```python
from build123d import *

# Parameters (mm, degrees)
SKETCH_1_W                = 48.5
SKETCH_1_H                = 37
EXTRUDE_1_DEPTH           = 3
SKETCH_2_W                = 21.920667416
SKETCH_2_H                = 2.787
CUT_EXTRUDE_1_DEPTH       = 32.646484797
SKETCH_6_W                = 21.920667416
SKETCH_6_H                = 2.787
CUT_EXTRUDE_5_DEPTH       = 32.646484797
EXTRUDE_2_DEPTH           = 3.028
EXTRUDE_3_DEPTH           = 3.028
HOLE_WIZARD_M4_1_D        = 4.447
HOLE_WIZARD_3_0_3_1_D     = 3
HOLE_WIZARD_3_0_3_1_DEPTH = 6.028
SKETCH_13_W               = 34.5
SKETCH_13_H               = 26.000497192
CUT_EXTRUDE_7_DEPTH       = 10
CHAMFER_1_SIZE            = 3
SKETCH_14_W               = 3
SKETCH_14_H               = 4
CUT_EXTRUDE_8_DEPTH       = 2
CHAMFER_2_SIZE            = 3
CHAMFER_2_SIZE_2          = 3.981134465
SKETCH_15_W               = 2
SKETCH_15_H               = 3
CUT_EXTRUDE_9_DEPTH       = 1.5
CHAMFER_3_SIZE            = 2


with BuildPart() as part:
    # 草图1 → 凸台-拉伸1 (new body)
    with BuildSketch(Plane.XY.offset(-11)):
        with Locations((1.25, 0)):
            Rectangle(SKETCH_1_W, SKETCH_1_H)
    extrude(amount=-EXTRUDE_1_DEPTH)

    # 草图2 → 切除-拉伸1 (cut, through all)
    with BuildSketch(Plane(origin=(0, 0, -14), x_dir=(-1, 0, 0), z_dir=(0, 0, -1))):
        with Locations((6.539666292, -11.606748596)):
            Rectangle(SKETCH_2_W, SKETCH_2_H)
    extrude(amount=-CUT_EXTRUDE_1_DEPTH, mode=Mode.SUBTRACT)

    # 草图6 → 切除-拉伸5 (cut, through all)
    with BuildSketch(Plane(origin=(0, 0, -14), x_dir=(-1, 0, 0), z_dir=(0, 0, -1))):
        with Locations((6.539666292, 11.606748596)):
            Rectangle(SKETCH_6_W, SKETCH_6_H)
    extrude(amount=-CUT_EXTRUDE_5_DEPTH, mode=Mode.SUBTRACT)

    # 草图7 → 凸台-拉伸2 (add)
    with BuildSketch(Plane.XY.offset(-11)):
        with BuildLine():
            Line((-20.5, -12), (-20.5, 12))
            ThreePointArc((-20.5, 12), (-19.914213562, 13.414213562), (-18.5, 14))
            Line((-18.5, 14), (-18.5, 12.914213562))
            ThreePointArc((-18.5, 12.914213562), (-19.224744871, 12.366025404), (-19.5, 11.5))
            Line((-19.5, 11.5), (-19.5, -11.5))
            ThreePointArc((-19.5, -11.5), (-19.224744871, -12.366025404), (-18.5, -12.914213562))
            Line((-18.5, -12.914213562), (-18.5, -14))
            ThreePointArc((-18.5, -14), (-19.914213562, -13.414213562), (-20.5, -12))
        make_face()
    extrude(amount=EXTRUDE_2_DEPTH)

    # 草图8 → 凸台-拉伸3 (add)
    with BuildSketch(Plane.XY.offset(-11)):
        with BuildLine():
            Line((19.5, -11.5), (19.5, 11.5))
            ThreePointArc((19.5, 11.5), (19.224744871, 12.366025404), (18.5, 12.914213562))
            Line((18.5, 12.914213562), (18.5, 14))
            ThreePointArc((18.5, 14), (19.914213562, 13.414213562), (20.5, 12))
            Line((20.5, 12), (20.5, -12))
            ThreePointArc((20.5, -12), (19.914213562, -13.414213562), (18.5, -14))
            Line((18.5, -14), (18.5, -12.914213562))
            ThreePointArc((18.5, -12.914213562), (19.224744871, -12.366025404), (19.5, -11.5))
        make_face()
    extrude(amount=EXTRUDE_3_DEPTH)

    # M4 间隙孔1 (through all)
    with Locations(Plane.XY.offset(-11)):
        with Locations((12.25, 6.000000304)):
            Hole(HOLE_WIZARD_M4_1_D / 2)

    # Ø3.0 (3) 直径孔1
    with Locations(Plane(origin=(0, 0, -14), x_dir=(-1, 0, 0), z_dir=(0, 0, -1))):
        with Locations((-15, -16.5), (15, -16.5), (0, -16.5), (-15, 16.5), (15, 16.5), (0, 16.5)):
            Hole(HOLE_WIZARD_3_0_3_1_D / 2, depth=HOLE_WIZARD_3_0_3_1_DEPTH)

    # 草图13 → 切除-拉伸7 (cut, symmetric)
    with BuildSketch(Plane(origin=(0, 0, -14), x_dir=(-1, 0, 0), z_dir=(0, 0, -1))):
        with Locations((0.75, 0)):
            Rectangle(SKETCH_13_W, SKETCH_13_H)
    extrude(amount=CUT_EXTRUDE_7_DEPTH, both=True, mode=Mode.SUBTRACT)

    # 倒角1
    chamfer_1_edges = [part.edges().sort_by_distance(p)[0] for p in [
        (-23, 18.5, -12.5),
        (25.5, 18.5, -12.5),
        (25.5, -18.5, -12.5),
        (-23, -18.5, -12.5),
    ]]
    chamfer(chamfer_1_edges, length=CHAMFER_1_SIZE)

    # 草图14 → 切除-拉伸8 (cut)
    with BuildSketch(Plane(origin=(0, 0, -14), x_dir=(-1, 0, 0), z_dir=(0, 0, -1))):
        with Locations((-7.5, -16.5)):
            Rectangle(SKETCH_14_W, SKETCH_14_H)
        with Locations((7.5, -16.5)):
            Rectangle(SKETCH_14_W, SKETCH_14_H)
        with Locations((7.5, 16.5)):
            Rectangle(SKETCH_14_W, SKETCH_14_H)
        with Locations((-7.5, 16.5)):
            Rectangle(SKETCH_14_W, SKETCH_14_H)
    extrude(amount=-CUT_EXTRUDE_8_DEPTH, mode=Mode.SUBTRACT)

    # 倒角2
    # the kernel refuses this chamfer: 3.981134465, 3 mm, written as the material it adds along each edge
    with BuildSketch(Plane(origin=(-6, 14.5, -12), x_dir=(0, -0.04104604510109815, -0.9991572559820394), z_dir=(-1, 0, 0))) as chamfer_2_piece_1_section:
        Polygon((CHAMFER_2_SIZE * 0.999157255982, -CHAMFER_2_SIZE * 0.0410460451011), (-CHAMFER_2_SIZE_2 * 0.0410460450997, -CHAMFER_2_SIZE_2 * 0.999157255947), (0, 0), align=None)
    chamfer_2_piece_1 = extrude(amount=3, mode=Mode.PRIVATE)
    chamfer_2_piece_1 = split(chamfer_2_piece_1, bisect_by=Plane(origin=(-7.5, 15.961237376, -14), z_dir=(0, 0, 1)), keep=Keep.TOP, mode=Mode.PRIVATE)
    add(chamfer_2_piece_1)
    with BuildSketch(Plane(origin=(9, 14.5, -12), x_dir=(0, -0.04104604510109815, -0.9991572559820394), z_dir=(-1, 0, 0))) as chamfer_2_piece_2_section:
        Polygon((CHAMFER_2_SIZE * 0.999157255982, -CHAMFER_2_SIZE * 0.0410460451011), (-CHAMFER_2_SIZE_2 * 0.0410460450997, -CHAMFER_2_SIZE_2 * 0.999157255947), (0, 0), align=None)
    chamfer_2_piece_2 = extrude(amount=3, mode=Mode.PRIVATE)
    chamfer_2_piece_2 = split(chamfer_2_piece_2, bisect_by=Plane(origin=(7.5, 15.961237376, -14), z_dir=(0, 0, 1)), keep=Keep.TOP, mode=Mode.PRIVATE)
    add(chamfer_2_piece_2)
    with BuildSketch(Plane(origin=(-9, -14.5, -12), x_dir=(0, -0.9997280272590685, 0.023321052992758363), z_dir=(1, 0, 0))) as chamfer_2_piece_3_section:
        Polygon((CHAMFER_2_SIZE_2 * 0.999728027224, CHAMFER_2_SIZE_2 * 0.0233210529919), (-CHAMFER_2_SIZE * 0.0233210529928, CHAMFER_2_SIZE * 0.999728027259), (0, 0), align=None)
    chamfer_2_piece_3 = extrude(amount=3, mode=Mode.PRIVATE)
    chamfer_2_piece_3 = split(chamfer_2_piece_3, bisect_by=Plane(origin=(-7.5, -15.961237376, -14), z_dir=(0, 0, 1)), keep=Keep.TOP, mode=Mode.PRIVATE)
    add(chamfer_2_piece_3)
    with BuildSketch(Plane(origin=(6, -14.5, -12), x_dir=(0, -0.9997280272590685, 0.023321052992758374), z_dir=(1, 0, 0))) as chamfer_2_piece_4_section:
        Polygon((CHAMFER_2_SIZE_2 * 0.999728027224, CHAMFER_2_SIZE_2 * 0.0233210529919), (-CHAMFER_2_SIZE * 0.0233210529928, CHAMFER_2_SIZE * 0.999728027259), (0, 0), align=None)
    chamfer_2_piece_4 = extrude(amount=3, mode=Mode.PRIVATE)
    chamfer_2_piece_4 = split(chamfer_2_piece_4, bisect_by=Plane(origin=(7.5, -15.961237376, -14), z_dir=(0, 0, 1)), keep=Keep.TOP, mode=Mode.PRIVATE)
    add(chamfer_2_piece_4)

    # 草图15 → 切除-拉伸9 (cut)
    with BuildSketch(Plane(origin=(0, 0, -14), x_dir=(-1, 0, 0), z_dir=(0, 0, -1))):
        with Locations((-24.5, -9.5)):
            Rectangle(SKETCH_15_W, SKETCH_15_H)
        with Locations((-24.5, 9.5)):
            Rectangle(SKETCH_15_W, SKETCH_15_H)
        with Locations((22, 9.5)):
            Rectangle(SKETCH_15_W, SKETCH_15_H)
        with Locations((22, -9.5)):
            Rectangle(SKETCH_15_W, SKETCH_15_H)
    extrude(amount=-CUT_EXTRUDE_9_DEPTH, mode=Mode.SUBTRACT)

    # 倒角3
    # the kernel refuses this chamfer: 2 mm, written as the material it adds along each edge
    with BuildSketch(Plane(origin=(-21, 2.856634024, -12.5), x_dir=(0.027495876610585623, 0, -0.9996219169112968), z_dir=(0, 1, 0))) as chamfer_3_piece_1_section:
        Polygon((CHAMFER_3_SIZE * 0.999621916911, CHAMFER_3_SIZE * 0.0274958766106), (-CHAMFER_3_SIZE * 0.0274958766106, CHAMFER_3_SIZE * 0.999621916911), (0, 0), align=None)
    chamfer_3_piece_1 = extrude(amount=13.286731952, mode=Mode.PRIVATE)
    chamfer_3_piece_1 = split(chamfer_3_piece_1, bisect_by=Plane(origin=(-21.7, 9.5, -14), z_dir=(0, 0, 1)), keep=Keep.TOP, mode=Mode.PRIVATE)
    chamfer_3_piece_1 = split(chamfer_3_piece_1, bisect_by=Plane(origin=(-25.35, 13.15, -13.1), z_dir=(0.7071067811865476, -0.7071067811865476, 0)), keep=Keep.TOP, mode=Mode.PRIVATE)
    add(chamfer_3_piece_1)
    with BuildSketch(Plane(origin=(-21, -2.856634024, -12.5), x_dir=(0.027495876610585623, 0, -0.9996219169112968), z_dir=(0, -1, 0))) as chamfer_3_piece_2_section:
        Polygon((CHAMFER_3_SIZE * 0.999621916911, -CHAMFER_3_SIZE * 0.0274958766106), (-CHAMFER_3_SIZE * 0.0274958766106, -CHAMFER_3_SIZE * 0.999621916911), (0, 0), align=None)
    chamfer_3_piece_2 = extrude(amount=8.143365976, mode=Mode.PRIVATE)
    chamfer_3_piece_2 = split(chamfer_3_piece_2, bisect_by=Plane(origin=(-21.7, -9.5, -14), z_dir=(0, 0, 1)), keep=Keep.TOP, mode=Mode.PRIVATE)
    add(chamfer_3_piece_2)
    with BuildSketch(Plane(origin=(23.5, 2.856634024, -12.5), x_dir=(-0.027495876610585623, 0, -0.9996219169112968), z_dir=(0, 1, 0))) as chamfer_3_piece_3_section:
        Polygon((CHAMFER_3_SIZE * 0.999621916911, -CHAMFER_3_SIZE * 0.0274958766106), (-CHAMFER_3_SIZE * 0.0274958766106, -CHAMFER_3_SIZE * 0.999621916911), (0, 0), align=None)
    chamfer_3_piece_3 = extrude(amount=8.143365976, mode=Mode.PRIVATE)
    chamfer_3_piece_3 = split(chamfer_3_piece_3, bisect_by=Plane(origin=(24.2, 9.5, -14), z_dir=(0, 0, 1)), keep=Keep.TOP, mode=Mode.PRIVATE)
    add(chamfer_3_piece_3)
    with BuildSketch(Plane(origin=(23.5, -2.856634024, -12.5), x_dir=(-0.027495876610585623, 0, -0.9996219169112968), z_dir=(0, -1, 0))) as chamfer_3_piece_4_section:
        Polygon((CHAMFER_3_SIZE * 0.999621916911, CHAMFER_3_SIZE * 0.0274958766106), (-CHAMFER_3_SIZE * 0.0274958766106, CHAMFER_3_SIZE * 0.999621916911), (0, 0), align=None)
    chamfer_3_piece_4 = extrude(amount=13.286731952, mode=Mode.PRIVATE)
    chamfer_3_piece_4 = split(chamfer_3_piece_4, bisect_by=Plane(origin=(24.2, -9.5, -14), z_dir=(0, 0, 1)), keep=Keep.TOP, mode=Mode.PRIVATE)
    chamfer_3_piece_4 = split(chamfer_3_piece_4, bisect_by=Plane(origin=(27.85, -13.15, -13.1), z_dir=(-0.7071067811865476, 0.7071067811865476, 0)), keep=Keep.TOP, mode=Mode.PRIVATE)
    add(chamfer_3_piece_4)


solid = part.part
```
Part model, mm, in its own coordinate system. A direction names the side the tool comes from. Give positions to 0.01 mm unless a question says otherwise; leave off trailing zeros. Loops run counter-clockwise (first coordinate to the right, second up) from the corner with the lowest first, then second, coordinate; pieces in that order, holes last. Notation, with made-up numbers: M -2,-31 L 28,-31 A24 ccw 28,-7 Z; hole C -32,27.25 d2. An arc over 180 degrees is marked long. Return JSON: item names as keys, results as strings.
1) 3-axis set-ups, long thin cutter, end or side, ignore diameter. For faces 4 (the face through (16.5, 0, -13)), 5 (the face through (24.9, 8, -13.4)), 6 (the face through (18.5, -13.5, -9.5)): which of +Z, -Z, +X, -X, +Y, -Y reach the whole face in a straight line?
Calculated:
{"face 4": "+Z, -Z", "face 5": "-Z, +X", "face 6": "+Z, +Y, -Y"}
2) Pull direction Y, two halves, no side cores. Call faces 1 (the face through (19.9, 13.43, -9.51)), 2 (the face through (-19.5, 0, -10)), 3 (the face through (20.5, 0, -10)): released by +Y, released by -Y, zero draft, split by the parting line, or undercut.
Calculated:
{"face 1": "released by +Y", "face 2": "undercut", "face 3": "zero draft"}
3) Saw through at D-D, the plane y = -16.5. List the corners of the cut face in (x, z).
Calculated:
{"outline": "M -22,-14 L -16.5,-14 L -16.5,-11 L -22,-11 Z; M -13.5,-14 L -9,-14 L -9,-13.49 L -6,-13.49 L -6,-14 L -1.5,-14 L -1.5,-11 L -13.5,-11 Z; M 1.5,-14 L 6,-14 L 6,-13.49 L 9,-13.49 L 9,-14 L 13.5,-14 L 13.5,-11 L 1.5,-11 Z; M 16.5,-14 L 24.5,-14 L 24.5,-11 L 16.5,-11 Z"}
4) Saw through at C-C, the plane z = -10. List the corners of the cut face in (x, y), then the cut area to 3 significant figures.
Calculated:
{"outline": "M -20.5,-12 A2 ccw -18.5,-14 L -18.5,-12.91 A1.5 cw -19.5,-11.5 L -19.5,11.5 A1.5 cw -18.5,12.91 L -18.5,14 A2 ccw -20.5,12 Z; M 18.5,-14 A2 ccw 20.5,-12 L 20.5,12 A2 ccw 18.5,14 L 18.5,12.91 A1.5 cw 19.5,11.5 L 19.5,-11.5 A1.5 cw 18.5,-12.91 Z", "area": "58.4 mm2"}
5) Drill centre lines: line 1 (Y direction, x = 0, z = -12.45); line 2 (X direction, y = 3.5, z = -10.75); line 3 (Y direction, x = -12.5, z = -13.5). Where is each one in solid material? Low to high.
Calculated:
{"line 1": "y = -18.5 to -18, -15 to -13, 13 to 15, 18 to 18.5", "line 2": "x = -20.5 to -19.5, 19.5 to 20.5", "line 3": "y = -18.5 to -13, 13 to 18.5"}
6) Saw through at A-A, the plane y = 6. List the corners of the cut face in (x, z).
Calculated:
{"outline": "M -23,-14 L -18,-14 L -18,-11 L -19.5,-11 L -19.5,-7.97 L -20.5,-7.97 L -20.5,-11 L -23,-11 Z; M 16.5,-14 L 25.5,-14 L 25.5,-11 L 20.5,-11 L 20.5,-7.97 L 19.5,-7.97 L 19.5,-11 L 16.5,-11 Z"}
7) Saw through at B-B, the plane x = -2. List the corners of the cut face in (y, z), then the cut area to 3 significant figures.
Calculated:
{"outline": "M -18.5,-14 L -13,-14 L -13,-11 L -18.5,-11 Z; M 13,-14 L 18.5,-14 L 18.5,-11 L 13,-11 Z", "area": "33.0 mm2"}
8) Flat gauge pins, fed straight in: pin 1 Ø0.6 at (y, z) = (16.5, -12.5) entering from -X; pin 2 Ø1.7 at (x, z) = (24.5, -13.5) entering from +Y; pin 3 Ø0.9 at (y, z) = (-13.5, -10) entering from +X; pin 4 Ø5 at (x, y) = (-16, 2) entering from -Z. Where does each tip first touch, or does it go through?
Calculated:
{"pin 1": "stops at x = -22.3", "pin 2": "stops at y = 17.35", "pin 3": "stops at x = 20.2", "pin 4": "stops at z = -14"}
